Part model, mm, in its own coordinate system. Give positions to 0.01 mm unless a question says otherwise; leave off trailing zeros. Write each loop counter-clockwise with the first axis right and the second up, starting at its lowest first coordinate (ties: lowest second). Pieces come first, ordered by that corner, then holes.
from build123d import *

# Parameters (mm, degrees)
BOSS_EXTRUDE1_DEPTH = 109.22
FILLET1_R           = 0.635
CHAMFER1_SIZE       = 5.08
SKETCH2_W           = 5.08
SKETCH2_H           = 1.397
BOSS_EXTRUDE2_DEPTH = 6.35


with BuildPart() as part:
    # Sketch1 → Boss-Extrude1 (new body)
    with BuildSketch(Plane.XY):
        with BuildLine():
            Line((24.4475, -5.7785), (-24.4475, -5.7785))
            ThreePointArc((-24.4475, -5.7785), (-30.226, 0), (-24.4475, 5.7785))
            Line((-24.4475, 5.7785), (24.4475, 5.7785))
            ThreePointArc((24.4475, 5.7785), (30.226, 0), (24.4475, -5.7785))
        make_face()
    extrude(amount=BOSS_EXTRUDE1_DEPTH)

    # Fillet1
    fillet1_edges = [part.edges().sort_by_distance(p)[0] for p in [
        (0, 5.7785, 0),
        (30.226, 0, 0),
        (0, -5.7785, 0),
        (-30.226, 0, 0),
    ]]
    fillet(fillet1_edges, radius=FILLET1_R)

    # Chamfer1
    # the kernel refuses this chamfer: 5.08 mm, written as the material it takes off along each edge
    with BuildSketch(Plane(origin=(-37.511649579, 5.7785, 109.22), x_dir=(0, 0.02749587661058642, -0.9996219169112968), z_dir=(1, 0, 0))) as chamfer1_piece_1:
        Polygon((CHAMFER1_SIZE * 0.999621916911, -CHAMFER1_SIZE * 0.0274958766106), (-CHAMFER1_SIZE * 0.0274958766106, -CHAMFER1_SIZE * 0.999621916911), (0, 0), align=None)
    extrude(amount=75.023299158, mode=Mode.SUBTRACT)
    with BuildSketch(Plane(origin=(37.511649579, -5.7785, 109.22), x_dir=(0, 0.9996219169112966, 0.02749587661058728), z_dir=(-1, 0, 0))) as chamfer1_piece_2:
        Polygon((CHAMFER1_SIZE * 0.999621916911, CHAMFER1_SIZE * 0.0274958766106), (-CHAMFER1_SIZE * 0.0274958766106, CHAMFER1_SIZE * 0.999621916911), (0, 0), align=None)
    extrude(amount=75.023299158, mode=Mode.SUBTRACT)

    # Sketch2 → Boss-Extrude2 (add)
    with BuildSketch(Plane.XY.offset(109.22)):
        with Locations((-16.51, 0)):
            Rectangle(SKETCH2_W, SKETCH2_H)
        with Locations((16.51, 0)):
            Rectangle(SKETCH2_W, SKETCH2_H)
    extrude(amount=BOSS_EXTRUDE2_DEPTH)


solid = part.part
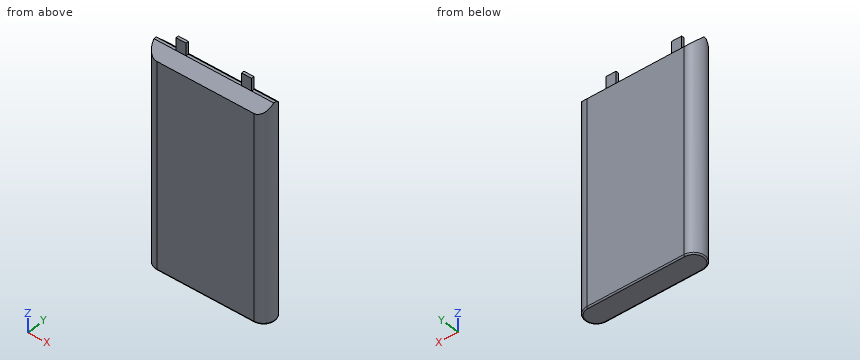
1) Flat gauge pins, fed straight in: P1, Ø1.5, axis at y = 0, z = 111.5, coming from the +X side; P2, Ø1.1, axis at x = 26.5, y = 0, coming from the +Z side; P3, Ø5.5, axis at x = 15.5, z = 113, coming from the -Y side. Where does each tip first touch, or does it go through?
Check result:
P1: stops at x = 19.05
P2: stops at z = 109.22
P3: stops at y = -0.7
2) Drill centre lines: L1, parallel to X at y = -0.75, z = 106; L2, parallel to Z at x = -27, y = -0.25; L3, parallel to Z at x = 4.5, y = -2.5. Where is each one in solid material? Low to high.
Check result:
L1: x = -30.18 to 30.18
L2: z = 0 to 109.22
L3: z = 0 to 107.42
3) Saw through at C-C (z = 106). Write the cut outline in (x, y).
Check result:
outline: (-28.69, -3.92) - (28.69, -3.92) arc R5.78 ccw to (28.69, 3.92) - (-28.69, 3.92) arc R5.78 ccw to start
4) Saw through at B-B (z = 88.5). Write the cut outline in (x, y).
Check result:
outline: (-24.45, -5.78) - (24.45, -5.78) arc R5.78 ccw to (24.45, 5.78) - (-24.45, 5.78) arc R5.78 ccw to start
5) Saw through at A-A (x = 1.5). Write the cut outline in (y, z) (1 decimal), and give its area (3 significant figures).
Check result:
outline: (-5.8, 0.6) arc R0.6 ccw to (-5.1, 0) - (5.1, 0) arc R0.6 ccw to (5.8, 0.6) - (5.8, 104.1) - (0.7, 109.2) - (-0.7, 109.2) - (-5.8, 104.1) - close
area: 1,240 mm2
